Could you check a few things on this drawing? It's one solid part, dimensions in mm from its lowest x, y, z. A direction names the side the tool comes from. Give positions to 0.01 mm unless a question says otherwise; leave off trailing zeros. Order: outer loops, then holes, each group sorted by start corner. A loop starts at its lowest first (then second) coordinate and runs counter-clockwise, first axis right, second up.
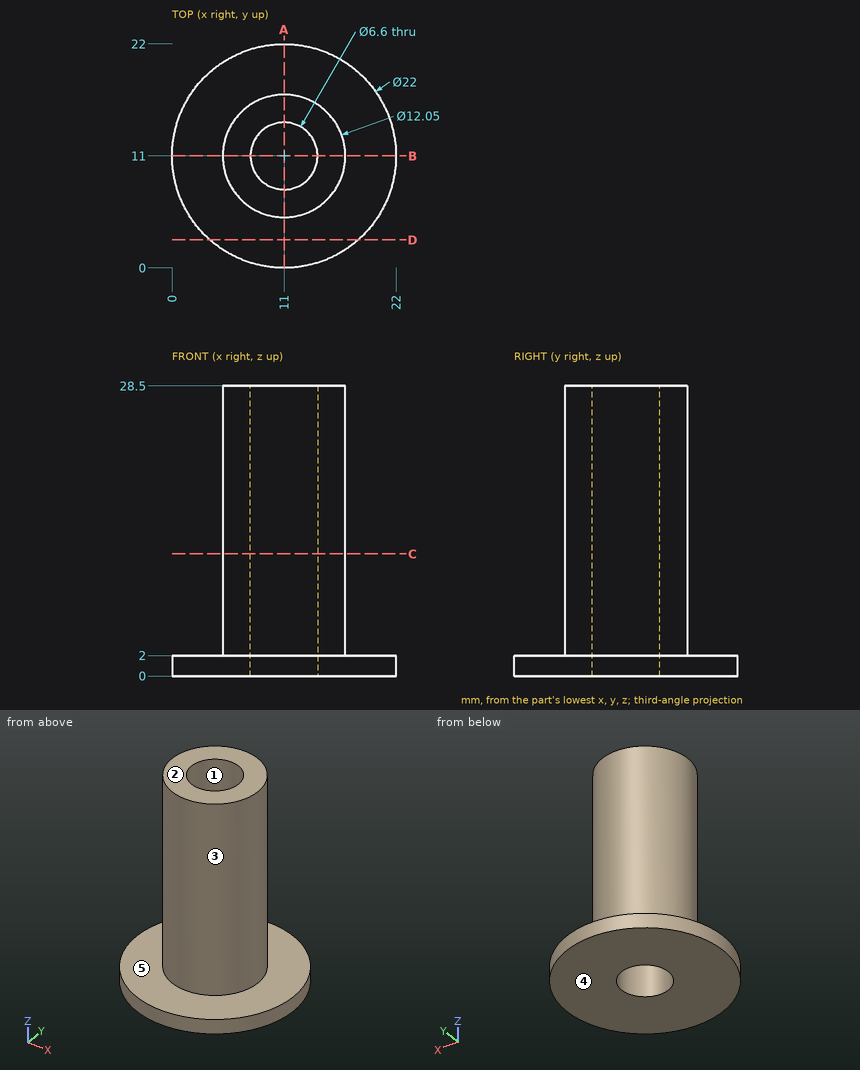
Item 1: Imagine slicing it at C-C on z = 12. List the corners of the cut face in (x, y) for me (3 decimals), then the cut area to 3 significant figures.
Findings:
outline: circle Ø12.05 at (11, 11); hole circle Ø6.6 at (11, 11)
area: 79.8 mm2
Item 2: Please list where these lines run through material, in increasing order: line 1 along Y through (x, z) = (11, 18.75) (3 decimals); line 2 along Z through (x, y) = (1, 14.75); line 3 along X through (y, z) = (9.5, 24.5).
Findings:
line 1: y = 4.975 to 7.7, 14.3 to 17.025
line 2: z = 0 to 2
line 3: x = 5.16 to 8.06, 13.94 to 16.84
Item 3: For the marked faces 4 and 5, which set-ups out of +Z, -Z, +X, -X, +Y, -Y let a thin tool reach every point of the face, with its end or its side?
Findings:
face 4: -Z, +X, -X, +Y, -Y
face 5: +Z
Item 4: Imagine slicing it at A-A on x = 11. List the corners of the cut face in (y, z) for me (3 decimals).
Findings:
outline: (0, 0) - (7.7, 0) - (7.7, 28.5) - (4.975, 28.5) - (4.975, 2) - (0, 2) - close; (14.3, 0) - (22, 0) - (22, 2) - (17.025, 2) - (17.025, 28.5) - (14.3, 28.5) - close
Item 5: We'd pull the mould along Y, two halves only. Please class the marked faces 1, 2 and 3: +Y half, -Y half, draft (parallel to the pull), parting line (faces both ways), or undercut.
Findings:
face 1: undercut
face 2: draft
face 3: parting line
Item 6: Imagine slicing it at D-D on y = 2.75. List the corners of the cut face in (x, z) for me.
Findings:
outline: (3.72, 0) - (18.28, 0) - (18.28, 2) - (3.72, 2) - close
Item 7: For pin 1 (2 mm diameter, centred on x = 11, y = 10, fed in from +Z); pin 2 (5 mm diameter, centred on x = 7, z = 16, fed in from -Y); pin 3 (6 mm diameter, centred on x = 13.5, z = 8, fed in from -Y) (3 decimals); pin 4 (3 mm diameter, centred on y = 16.5, z = 20, fed in from +X), each with a flat end and sliding along its axis, tell me the tip position at first contact or that it passes through.
Findings:
pin 1: passes through
pin 2: stops at y = 5.16
pin 3: stops at y = 4.975
pin 4: stops at x = 15.51
